CAD build for the part. Positions are in the model's coordinates, mm. A direction names the side the tool comes from. Give positions to 0.01 mm unless a question says otherwise; leave off trailing zeros. Loops run counter-clockwise (first coordinate to the right, second up) from the corner with the lowest first, then second, coordinate; pieces in that order, holes last.
```python
from build123d import *

# Parameters (mm, degrees)
F0_W     = 25
F0_H     = 24
F1_DEPTH = 7.62
F2_R     = 4
F3_DEPTH = 6.35
F4_R     = 4.8022038817
F4_R_2   = 4
F5_DEPTH = 1
F6_SIZE  = 2.54
F7_R     = 1.905
F8_R     = 4.8792946489
F9_DEPTH = 5.08
F10_R    = 1.27


with BuildPart() as f1:
    # F0 (on Top) → F1 (new body)
    with BuildSketch(Plane.XY):
        with Locations((12.5, 12)):
            Rectangle(F0_W, F0_H)
    extrude(amount=F1_DEPTH)

    # F2 (on face) → F3 (join)
    with BuildSketch(Plane.XY.offset(7.62)):
        with Locations((15.5, 12.2524611652)):
            Circle(F2_R)
    extrude(amount=F3_DEPTH)

    # F4 (on face) → F5 (join)
    with BuildSketch(Plane.XY.offset(13.97)):
        with Locations((15.5, 12.2524611652)):
            Circle(F4_R)
        with Locations((15.5, 12.2524611652)):
            Circle(F4_R_2, mode=Mode.SUBTRACT)
        with Locations((15.5, 12.2524611652)):
            Circle(F4_R_2)
    extrude(amount=F5_DEPTH)

    # F6
    f6_edges = [f1.edges().sort_by_distance(p)[0] for p in [
        (0, 12, 7.62),
        (12.5, 24, 7.62),
        (12.5, 0, 7.62),
        (25, 12, 7.62),
        (11.5, 12.252461, 7.62),
    ]]
    chamfer(f6_edges, length=F6_SIZE)

    # F7
    f7_edges = [f1.edges().sort_by_distance(p)[0] for p in [
        (0, 12, 0),
        (12.5, 0, 0),
        (25, 12, 0),
        (12.5, 24, 0),
        (25, 24, 2.54),
        (25, 0, 2.54),
        (0, 0, 2.54),
        (0, 24, 2.54),
    ]]
    fillet(f7_edges, radius=F7_R)

    # F8 (on face) → F9 (join)
    with BuildSketch(Plane(origin=(0, 0, 0), x_dir=(1, 0, 0), z_dir=(0, 0, -1))):
        with Locations((12.7, -12)):
            Circle(F8_R)
    extrude(amount=F9_DEPTH)

    # F10
    f10_edges = [f1.edges().sort_by_distance(p)[0] for p in [
        (7.820705, 12, -5.08),
    ]]
    fillet(f10_edges, radius=F10_R)


solid = f1.part
```
1. Saw through at A-A, the plane x = 4. List the corners of the cut face in (y, z) (3 decimals), and give its area (3 significant figures).
Responses:
outline: (0, 1.905) arc R1.905 ccw to (1.905, 0) - (22.095, 0) arc R1.905 ccw to (24, 1.905) - (24, 5.08) - (21.46, 7.62) - (2.54, 7.62) - (0, 5.08) - close
area: 175 mm2
2. Probe line 1 along Z through (x, y) = (17.75, 12.5); line 2 along Z through (x, y) = (12, 6); line 3 along Y through (x, z) = (7, 1.75). List the from-to ranges inside material, lowest first.
Responses:
line 1: z = 0 to 14.97
line 2: z = 0 to 7.62
line 3: y = 0.01 to 23.99
3. Saw through at B-B, the plane z = 1.25. List the corners of the cut face in (x, y) (3 decimals), and give its area (3 significant figures).
Responses:
outline: (0.116, 1.905) arc R1.789 ccw to (1.905, 0.116) - (23.095, 0.116) arc R1.789 ccw to (24.884, 1.905) - (24.884, 22.095) arc R1.789 ccw to (23.095, 23.884) - (1.905, 23.884) arc R1.789 ccw to (0.116, 22.095) - close
area: 586 mm2
4. Tool access for faces 4 (the face through (12, 0, 3)), 5 (the face through (17.207, 13.869, -1.878)), 6 (the face through (8, 12, 7.62)): list every direction of +Z, -Z, +X, -X, +Y, -Y with a clear straight run to the whole face (end or side of a thin tool).
Responses:
face 4: +Z, -Z, +X, -X, -Y
face 5: -Z
face 6: +Z
5. Drop flat-ended pins along their axis: pin 1 (1.5 mm diameter, centred on x = 8, y = 11, fed in from +Z); pin 2 (6 mm diameter, centred on x = 3, y = 19, fed in from -Z); pin 3 (5 mm diameter, centred on x = 7, z = -0.5, fed in from -Y). Give the stop position or say it passes through.
Responses:
pin 1: stops at z = 7.62
pin 2: stops at z = 0
pin 3: stops at y = 0
6. Pull direction Z, two halves, no side cores. Call faces 1 (the face through (7.6, 12.1, 0)), 2 (the face through (17.74, 15.76, 10)), 3 (the face through (19.936, 10.413, 14.463)): released by +Z, released by -Z, zero draft, split by the parting line, or undercut.
Responses:
face 1: released by -Z
face 2: undercut
face 3: zero draft
7. Saw through at C-C, the plane z = -2.5. List the corners of the cut face in (x, y).
Responses:
outline: circle Ø9.76 at (12.7, 12)
